Geometry check sheet. Reference: drawing and pictorial views, mm from the part's lowest x, y, z. Give positions to 0.01 mm unless a question says otherwise; leave off trailing zeros. Write each loop counter-clockwise with the first axis right and the second up, starting at its lowest first coordinate (ties: lowest second). Pieces come first, ordered by that corner, then holes.
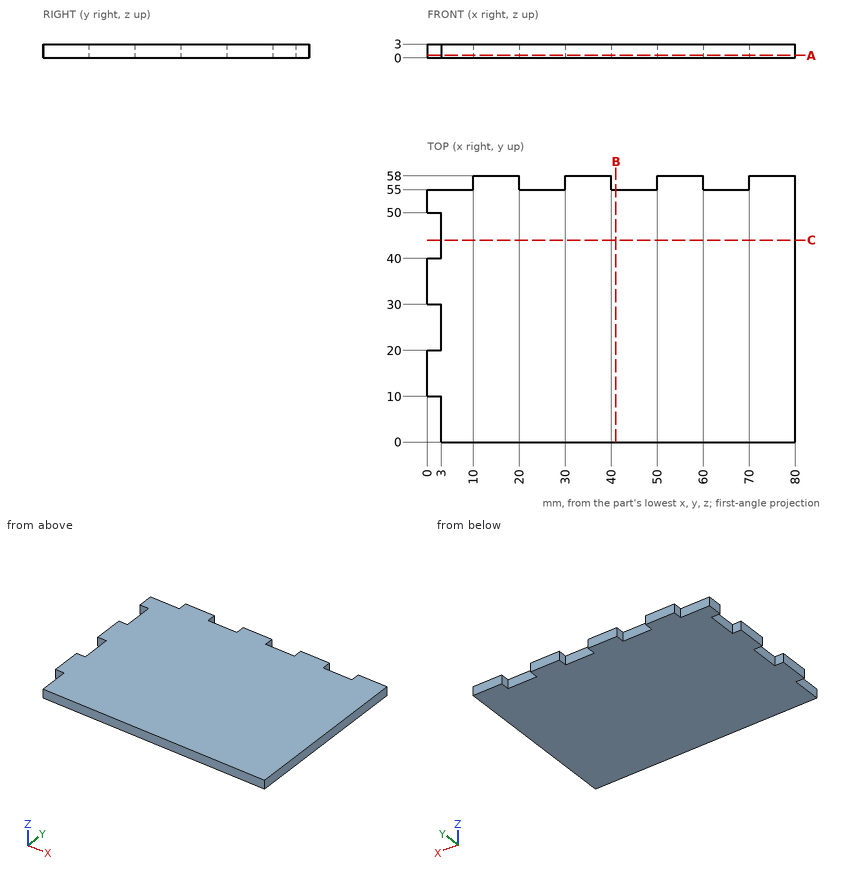
Item 1: Sectioned sample at B-B on x = 41. Record the cut outline in (y, z), then the cut area to 3 significant figures.
Answer key:
outline: (0, 0) - (55, 0) - (55, 3) - (0, 3) - close
area: 165 mm2
Item 2: Sectioned sample at C-C on y = 44. Record the cut outline in (x, z).
Answer key:
outline: (3, 0) - (80, 0) - (80, 3) - (3, 3) - close
Item 3: Sectioned sample at A-A on z = 0.5. Record the cut outline in (x, y).
Answer key:
outline: (0, 10) - (3, 10) - (3, 0) - (80, 0) - (80, 58) - (70, 58) - (70, 55) - (60, 55) - (60, 58) - (50, 58) - (50, 55) - (40, 55) - (40, 58) - (30, 58) - (30, 55) - (20, 55) - (20, 58) - (10, 58) - (10, 55) - (0, 55) - (0, 50) - (3, 50) - (3, 40) - (0, 40) - (0, 30) - (3, 30) - (3, 20) - (0, 20) - close
Item 4: Depth check by flat-ended pin: pin 1 (0.9 mm diameter, centred on y = 46, z = 1, fed in from -X); pin 2 (1.5 mm diameter, centred on y = 56.5, z = 2, fed in from -X); pin 3 (0.9 mm diameter, centred on x = 1.5, z = 1, fed in from -Y). Enter the tip coordinate at first touch or a pass-through.
Answer key:
pin 1: stops at x = 3
pin 2: stops at x = 10
pin 3: stops at y = 10
Item 5: Scan lines: line 1 along X through (y, z) = (41.5, 2.35); line 2 along Y through (x, z) = (25, 0.9). Record each from-to range of solid material in increasing order.
Answer key:
line 1: x = 3 to 80
line 2: y = 0 to 55
